from build123d import *
from build123d.topology import SkipClean

# Parameters (mm, degrees)
CROQUIS1_W                = 15
CROQUIS1_H                = 10
CROQUIS1_R                = 1.6
SALIENTE_EXTRUIR2_DEPTH   = 25
SALIENTE_EXTRUIR2_2_DEPTH = 25
CROQUIS1_W_2              = 10
SALIENTE_EXTRUIR2_3_DEPTH = 25
SALIENTE_EXTRUIR2_4_DEPTH = 25
SALIENTE_EXTRUIR3_START   = 4
CROQUIS2_R                = 1.6
CROQUIS2_W                = 15
CROQUIS2_H                = 10
SALIENTE_EXTRUIR3_DEPTH   = 4
CROQUIS3_W                = 15
CROQUIS3_H                = 4
CROQUIS3_W_2              = 10
SALIENTE_EXTRUIR4_DEPTH   = 15
CROQUIS4_R                = 3.5
CORTAR_EXTRUIR1_DEPTH     = 3.5
SALIENTE_EXTRUIR5_DEPTH   = 3
CROQUIS6_R                = 1.6
CORTAR_EXTRUIR2_DEPTH     = 3
CORTAR_EXTRUIR3_DEPTH     = 1.5
REDONDEO1_R               = 2


with BuildPart() as part:
    # Croquis1 → Saliente-Extruir2 (new body)
    with BuildSketch(Plane(origin=(0, 0, 0), x_dir=(1, 0, 0), z_dir=(0, 1, 0))):
        with Locations((-17.954545455, 17.15034965)):
            Rectangle(CROQUIS1_W, CROQUIS1_H)
        with Locations(Location((-17.954545455, 17.15034965, 0), (0, 0, 270))):
            Circle(CROQUIS1_R, mode=Mode.SUBTRACT)
    extrude(amount=SALIENTE_EXTRUIR2_DEPTH)



with BuildPart() as body_2:
    # Croquis1 → Saliente-Extruir2 2 (new body)
    with BuildSketch(Plane(origin=(0, 0, 0), x_dir=(1, 0, 0), z_dir=(0, 1, 0))):
        with Locations((-17.954545455, -42.84965035)):
            Rectangle(CROQUIS1_W, CROQUIS1_H)
        with Locations(Location((-17.954545455, -42.84965035, 0), (0, 0, 270))):
            Circle(CROQUIS1_R, mode=Mode.SUBTRACT)
    extrude(amount=SALIENTE_EXTRUIR2_2_DEPTH)


with BuildPart() as body_3:
    # Croquis1 → Saliente-Extruir2 3 (new body)
    with BuildSketch(Plane(origin=(0, 0, 0), x_dir=(1, 0, 0), z_dir=(0, 1, 0))):
        with Locations((39.545454545, -42.84965035)):
            Rectangle(CROQUIS1_W_2, CROQUIS1_H)
        with Locations(Location((39.545454545, -42.84965035, 0), (0, 0, 270))):
            Circle(CROQUIS1_R, mode=Mode.SUBTRACT)
    extrude(amount=SALIENTE_EXTRUIR2_3_DEPTH)


with BuildPart() as body_4:
    # Croquis1 → Saliente-Extruir2 4 (new body)
    with BuildSketch(Plane(origin=(0, 0, 0), x_dir=(1, 0, 0), z_dir=(0, 1, 0))):
        with Locations((39.545454545, 17.15034965)):
            Rectangle(CROQUIS1_W_2, CROQUIS1_H)
        with Locations(Location((39.545454545, 17.15034965, 0), (0, 0, 270))):
            Circle(CROQUIS1_R, mode=Mode.SUBTRACT)
    extrude(amount=SALIENTE_EXTRUIR2_4_DEPTH)


with BuildPart() as part_1:
    with SkipClean():  # the faces are left unmerged after this step: merging them gives an invalid solid
        add(part.part)

        add(body_2.part)  # Saliente-Extruir3 merges body 2

        add(body_3.part)  # Saliente-Extruir3 merges body 3

        add(body_4.part)  # Saliente-Extruir3 merges body 4
        # Croquis2 → Saliente-Extruir3 (add)
        # profile 1 of 3: a face of its own
        with BuildSketch(Plane.XZ.offset(SALIENTE_EXTRUIR3_START)):
            Polygon((-25.454545455, -22.15034965), (-10.454545455, -22.15034965), (-10.454545455, -12.15034965), (-10.454545455, 37.84965035), (-25.454545455, 37.84965035), (-25.454545455, -12.15034965), align=None)
            with Locations(Location((-17.954545455, -17.15034965, 0), (0, 0, 270))):
                Circle(CROQUIS2_R, mode=Mode.SUBTRACT)
        # profile 2 of 3: a face of its own
        with BuildSketch(Plane.XZ.offset(SALIENTE_EXTRUIR3_START)):
            with Locations((-17.954545455, 42.84965035)):
                Rectangle(CROQUIS2_W, CROQUIS2_H)
            with Locations(Location((-17.954545455, 42.84965035, 0), (0, 0, 90))):
                Circle(CROQUIS2_R, mode=Mode.SUBTRACT)
        # profile 3 of 3: a face of its own
        with BuildSketch(Plane.XZ.offset(SALIENTE_EXTRUIR3_START)):
            Polygon((34.545454545, -12.15034965), (34.545454545, -22.15034965), (44.545454545, -22.15034965), (44.545454545, -12.15034965), (44.545454545, 37.84965035), (44.545454545, 47.84965035), (34.545454545, 47.84965035), (34.545454545, 37.84965035), align=None)
            with Locations(Location((39.545454545, -17.15034965, 0), (0, 0, 90))):
                Circle(CROQUIS2_R, mode=Mode.SUBTRACT)
            with Locations(Location((39.545454545, 42.84965035, 0), (0, 0, 270))):
                Circle(CROQUIS2_R, mode=Mode.SUBTRACT)
        extrude(amount=-SALIENTE_EXTRUIR3_DEPTH)

    # Croquis3 → Saliente-Extruir4 (add)
    with BuildSketch(Plane(origin=(0, 0, 0), x_dir=(1, 0, 0), z_dir=(0, 1, 0))):
        with Locations((-17.954545455, -35.84965035)):
            Rectangle(CROQUIS3_W, CROQUIS3_H)
        with Locations((-17.954545455, 10.15034965)):
            Rectangle(CROQUIS3_W, CROQUIS3_H)
        with Locations((39.545454545, 10.15034965)):
            Rectangle(CROQUIS3_W_2, CROQUIS3_H)
        with Locations((39.545454545, -35.84965035)):
            Rectangle(CROQUIS3_W_2, CROQUIS3_H)
    extrude(amount=SALIENTE_EXTRUIR4_DEPTH)

    # Croquis4 → Cortar-Extruir1 (cut)
    with SkipClean():  # the faces are left unmerged after this step: merging them gives an invalid solid
        with BuildSketch(Plane.XZ.offset(4)):
            with Locations(Location((39.545454545, 42.84965035, 0), (0, 0, 270))):
                Circle(CROQUIS4_R)
            with Locations(Location((39.545454545, -17.15034965, 0), (0, 0, 270))):
                Circle(CROQUIS4_R)
            with Locations(Location((-17.954545455, -17.15034965, 0), (0, 0, 270))):
                Circle(CROQUIS4_R)
            with Locations(Location((-17.954545455, 42.84965035, 0), (0, 0, 270))):
                Circle(CROQUIS4_R)
        extrude(amount=-CORTAR_EXTRUIR1_DEPTH, mode=Mode.SUBTRACT)

    # Croquis5 → Saliente-Extruir5 (add)
    with SkipClean():  # the faces are left unmerged after this step: merging them gives an invalid solid
        with BuildSketch(Plane.XZ.offset(4)):
            Polygon((-10.454545455, 40.07981816), (34.545454545, 40.07981816), (34.545454545, 35.84965035), (34.545454545, 28.84965035), (-10.454545455, 28.84965035), (-10.454545455, 35.84965035), align=None)
        extrude(amount=-SALIENTE_EXTRUIR5_DEPTH)

    # Croquis6 → Cortar-Extruir2 (cut)
    with SkipClean():  # the faces are left unmerged after this step: merging them gives an invalid solid
        with BuildSketch(Plane.XZ.offset(4)):
            with Locations(Location((24.045454545, 34.84965035, 0), (0, 0, 270))):
                Circle(CROQUIS6_R)
            with Locations(Location((0.045454545, 34.84965035, 0), (0, 0, 270))):
                Circle(CROQUIS6_R)
        extrude(amount=-CORTAR_EXTRUIR2_DEPTH, mode=Mode.SUBTRACT)

    # Croquis7 → Cortar-Extruir3 (cut)
    with SkipClean():  # the faces are left unmerged after this step: merging them gives an invalid solid
        with BuildSketch(Plane(origin=(0, -1, 0), x_dir=(1, 0, 0), z_dir=(0, 1, 0))):
            Polygon((0.045454545, -31.0968736), (-3.204545455, -32.973261975), (-3.204545455, -36.726038725), (0.045454545, -38.602427099), (3.295454545, -36.726038725), (3.295454545, -32.973261975), align=None)
            Polygon((24.045454545, -31.0968736), (20.795454545, -32.973261975), (20.795454545, -36.726038725), (24.045454545, -38.602427099), (27.295454545, -36.726038725), (27.295454545, -32.973261975), align=None)
        extrude(amount=-CORTAR_EXTRUIR3_DEPTH, mode=Mode.SUBTRACT)

    # Redondeo1
    # the kernel refuses this fillet: 2 mm, written as the material it takes off along each edge
    with BuildSketch(Plane(origin=(-5.454545455, -4, 47.84965035), x_dir=(0, 0, -1), z_dir=(-1, 0, 0)), Plane(origin=(-30.454545455, -4, -22.15034965), x_dir=(0, 0, 1), z_dir=(1, 0, 0))) as redondeo1_piece_1:
        with BuildLine():
            CenterArc((REDONDEO1_R, -REDONDEO1_R), REDONDEO1_R, 90, 90)
            Line((0, -REDONDEO1_R), (0, 0))
            Line((0, 0), (REDONDEO1_R, 0))
        make_face()
    extrude(amount=25, mode=Mode.SUBTRACT)
    with BuildSketch(Plane(origin=(29.545454545, -4, -22.15034965), x_dir=(0, 1, 0), z_dir=(1, 0, 0))) as redondeo1_piece_2:
        with BuildLine():
            CenterArc((REDONDEO1_R, REDONDEO1_R), REDONDEO1_R, 180, 90)
            Line((0, REDONDEO1_R), (0, 0))
            Line((0, 0), (REDONDEO1_R, 0))
        make_face()
    extrude(amount=20, mode=Mode.SUBTRACT)


solid = part_1.part
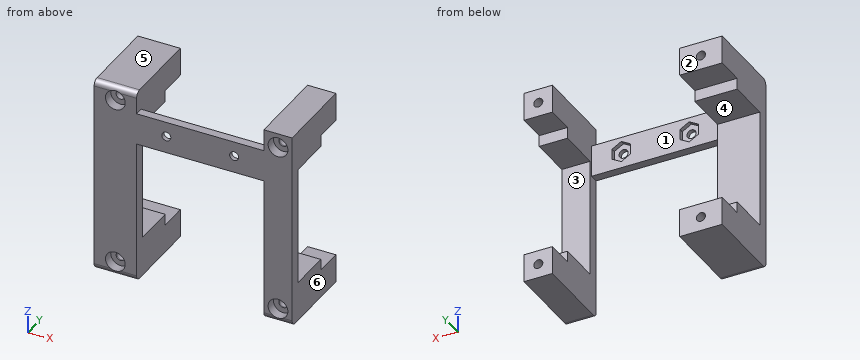
Verification items for the finished model (mm, model axes). Face numbers are marked on the shaded views. A direction names the side the tool comes from. Give positions to 0.01 mm unless a question says otherwise; leave off trailing zeros. Write each loop counter-clockwise with the first axis right and the second up, starting at its lowest first coordinate (ties: lowest second). Pieces come first, ordered by that corner, then holes.
(1) Gauge pin test, flat ends, axial feed: pin 1 (5.5 mm diameter, centred on x = 40, z = 43.5, fed in from -Y); pin 2 (3.5 mm diameter, centred on x = -17.5, z = -15.5, fed in from -Y); pin 3 (3 mm diameter, centred on x = 24, z = 34, fed in from +Y); pin 4 (7 mm diameter, centred on x = 0.5, z = 34, fed in from +Y). Record the tip position at first contact, or that the pin passes through.
(2) Access from +Z, -Z, +X, -X, +Y, -Y to the whole of each face (thin tool, end or side, straight path). Record for the marked faces 1, 2 and 3.
(3) Material ranges on line 1 (Z direction, x = 36, y = 10.25); line 2 (Z direction, x = 39, y = 22.75); line 3 (X direction, y = -1.5, z = -19), recorded low to high.
(4) Cross-section at D-D (x = 7.5). Enter the section's corners in (y, z).
(5) Cross-section at C-C (y = 19). Enter the section's corners in (x, z).
(6) Cross-section at A-A (z = -9). Enter the section's corners in (x, y), plus the area to 3 significant figures.
(7) Mould release check, pull along Z, two halves, no side actions. Record for the marked faces 4, 5 and 6: +Z half, -Z half, draft (parallel to the pull), parting line (faces both ways), or undercut.
(8) Cross-section at B-B (y = 5). Enter the section's corners in (x, z), plus the area to 3 significant figures.
Worked out:
1. pin 1: stops at y = -4
1. pin 2: stops at y = -0.5
1. pin 3: stops at y = -2.5
1. pin 4: stops at y = -1
2. face 1: +Z, -Z, +Y
2. face 2: +Z, -Z, +X, -X, +Y
2. face 3: +X, -X, +Y
3. line 1: z = -22.15 to -8.15, 33.85 to 47.85
3. line 2: z = -22.15 to -18.65, -15.65 to -12.15, 37.85 to 41.35, 44.35 to 47.85
3. line 3: x = -25.45 to -20.93, -14.98 to -10.45, 34.55 to 36.57, 42.52 to 44.55
4. outline: (-4, 28.85) - (-1, 28.85) - (-1, 40.08) - (-4, 40.08) - close
5. outline: (-25.45, -22.15) - (-10.45, -22.15) - (-10.45, -12.15) - (-25.45, -12.15) - close; (-25.45, 37.85) - (-10.45, 37.85) - (-10.45, 47.85) - (-25.45, 47.85) - close; (34.55, -22.15) - (44.55, -22.15) - (44.55, -12.15) - (34.55, -12.15) - close; (34.55, 37.85) - (44.55, 37.85) - (44.55, 47.85) - (34.55, 47.85) - close; hole circle Ø3.2 at (-17.95, -17.15); hole circle Ø3.2 at (-17.95, 42.85); hole circle Ø3.2 at (39.55, -17.15); hole circle Ø3.2 at (39.55, 42.85)
6. outline: (-25.45, -4) - (-10.45, -4) - (-10.45, 15) - (-25.45, 15) - close; (34.55, -4) - (44.55, -4) - (44.55, 15) - (34.55, 15) - close
6. area: 475 mm2
7. face 4: undercut
7. face 5: +Z half
7. face 6: draft
8. outline: (-25.45, -22.15) - (-10.45, -22.15) - (-10.45, -8.15) - (-25.45, -8.15) - close; (-25.45, 33.85) - (-10.45, 33.85) - (-10.45, 47.85) - (-25.45, 47.85) - close; (34.55, -22.15) - (44.55, -22.15) - (44.55, -8.15) - (34.55, -8.15) - close; (34.55, 33.85) - (44.55, 33.85) - (44.55, 47.85) - (34.55, 47.85) - close; hole circle Ø3.2 at (-17.95, -17.15); hole circle Ø3.2 at (-17.95, 42.85); hole circle Ø3.2 at (39.55, -17.15); hole circle Ø3.2 at (39.55, 42.85)
8. area: 668 mm2
